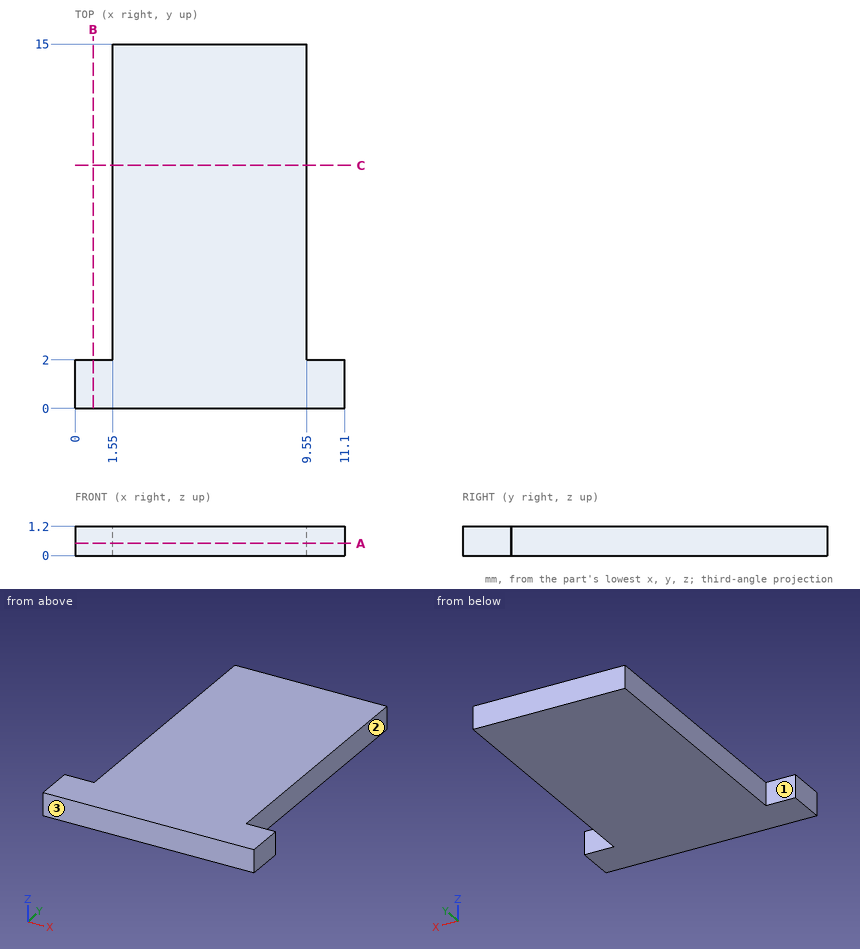
Job drawing, mm, ordinate dimensions from the low corner. One solid piece. A direction names the side the tool comes from. Coordinates: 2 decimals unless noted, no trailing zeros. Write each loop counter-clockwise with the first axis right and the second up, starting at its lowest first coordinate (ties: lowest second). Pieces come first, ordered by that corner, then holes.
Item 1: Slice it at C-C (y = 10). Write the cut outline in (x, z).
Item 2: Probe line 1 (X direction, y = 12, z = 0.4); line 2 (Y direction, x = 0.5, z = 0.9). List the from-to ranges inside material, lowest first.
Item 3: Slice it at A-A (z = 0.5). Write the cut outline in (x, y).
Item 4: Slice it at B-B (x = 0.75). Write the cut outline in (y, z).
Item 5: Which spindle directions (+Z, -Z, +X, -X, +Y, -Y) get a long thin tool onto all of the face, cutting with end or side? Do the marked faces 1, 2 and 3. Say none if no direction does.
Item 6: Pin check, flat tip, straight feed: pin 1 (0.6 mm diameter, centred on y = 9, z = 1, fed in from -X). Stop position of the tip, or through.
Results found:
1. outline: (1.55, 0) - (9.55, 0) - (9.55, 1.2) - (1.55, 1.2) - close
2. line 1: x = 1.55 to 9.55
2. line 2: y = 0 to 2
3. outline: (0, 0) - (11.1, 0) - (11.1, 2) - (9.55, 2) - (9.55, 15) - (1.55, 15) - (1.55, 2) - (0, 2) - close
4. outline: (0, 0) - (2, 0) - (2, 1.2) - (0, 1.2) - close
5. face 1: +Z, -Z, -X, +Y
5. face 2: +Z, -Z, +X, +Y
5. face 3: +Z, -Z, +X, -X, -Y
6. pin 1: stops at x = 1.55
